Work out the finished part from the listing and answer in its coordinate system (mm). Face numbers are marked on the shaded views. A direction names the side the tool comes from. Coordinates: 2 decimals unless noted, no trailing zeros. Order: outer loops, then holes, each group sorted by start corner. A loop starts at its lowest first (then second) coordinate and runs counter-clockwise, first axis right, second up.
1. Find the intervals of material crossed by probe 1 along X at (y, z) = (104.5, 44.5); probe 2 along Y at (x, z) = (-40, -46); probe 3 along X at (y, z) = (10.5, 18.5), in increasing order.
2. The part is cut by section C-C, the plane x = 41. Give the vertices of the cut face in (y, z), then the cut area to 3 significant figures.
3. The part is cut by section B-B, the plane z = -39. Give the vertices of the cut face in (x, y), then the cut area to 3 significant figures.
4. A tool of negligible diameter and unlimited length cuts with its end or side. For the marked faces 4, 5, 6 and 7, from which of +Z, -Z, +X, -X, +Y, -Y can it reach the whole face along a straight path? Write none if from no direction.
5. Determine the mould class of the marked faces 1, 2 and 3 for opening direction X: +X half, -X half, draft (parallel to the pull), parting line (faces both ways), or undercut.
6. Flat-ended cylindrical pins translate along their axes: pin 1 Ø13 at (x, z) = (34.5, -22) entering from +Y; pin 2 Ø1 at (y, z) = (61, 24.5) entering from +X; pin 3 Ø10 at (y, z) = (75, 26) entering from -X. Find the tip coordinate at first contact, or state that the pin passes through.
7. The part is cut by section A-A, the plane y = 16.5. Give the vertices of the cut face in (x, z).
Autodesk Fusion 360 part; units mm, degrees
sketch "Esquisse1" plane through (0, 0, 0) normal (0, 0, 1) x (1, 0, 0)
  line L0 (0, 10) -> (-12.5, 10)
  line L1 (-12.5, 10) -> (-12.5, 110)
  line L2 (-12.5, 110) -> (-22.5, 110)
  line L3 (-22.5, 110) -> (-22.5, 10)
  line L4 (-22.5, 10) -> (-55.5, 10)
  line L5 (-55.5, 10) -> (-55.5, 0)
  line L6 (-55.5, 0) -> (0, 0)
  line L7 (0, 1.75) -> (0, 22.5)
  line L8 (1.75, 0) -> (22.5, 0)
  line L9 (0, 10) -> (12.5, 10)
  line L10 (12.5, 10) -> (12.5, 110)
  line L11 (12.5, 110) -> (22.5, 110)
  line L12 (22.5, 110) -> (22.5, 10)
  line L13 (22.5, 10) -> (55.5, 10)
  line L14 (55.5, 10) -> (55.5, 0)
  line L15 (55.5, 0) -> (0, 0)
  dimension "d13" = 12.5
  dimension "d15" = 10
  dimension "d16" = 10
  dimension "d17" = 100
  dimension "d19" = 10
  dimension "d20" = 55.5
extrude "Extrusion1" add sketch "Esquisse1" along normal mid plane 100
fillet "Congé5" radius 1.5 1 edges at (55.5, 10, 0)
fillet "Congé5" radius 1.5 1 edges at (-55.5, 10, 0)
fillet "Congé5" radius 1.5 1 edges at (12.5, 10, 0)
fillet "Congé5" radius 1.5 1 edges at (-12.5, 10, 0)
fillet "Congé5" radius 1.5 1 edges at (0, 10, -50)
fillet "Congé5" radius 1.5 1 edges at (0, 10, 50)
fillet "Congé6" radius 5 1 edges at (22.5, 10, 0)
fillet "Congé6" radius 5 1 edges at (-22.5, 10, 0)
fillet "Congé7" radius 1.5 5 edges at (-22.5, 62.5, 50) (-23.9645, 11.4645, 50) (-40.75, 10, 50) (-55.0607, 9.5607, 50) (-55.5, 4.25, 50)
fillet "Congé7" radius 1.5 5 edges at (22.5, 62.5, 50) (23.9645, 11.4645, 50) (40.75, 10, 50) (55.0607, 9.5607, 50) (55.5, 4.25, 50)
fillet "Congé7" radius 1.5 5 edges at (-55.5, 4.25, -50) (-55.0607, 9.5607, -50) (-40.75, 10, -50) (-23.9645, 11.4645, -50) (-22.5, 62.5, -50)
fillet "Congé7" radius 1.5 5 edges at (22.5, 62.5, -50) (23.9645, 11.4645, -50) (40.75, 10, -50) (55.0607, 9.5607, -50) (55.5, 4.25, -50)
fillet "Congé7" radius 1.5 1 edges at (17.5, 110, 50)
fillet "Congé7" radius 1.5 1 edges at (-17.5, 110, 50)
fillet "Congé7" radius 1.5 1 edges at (-17.5, 110, -50)
fillet "Congé7" radius 1.5 1 edges at (17.5, 110, -50)
fillet "Congé7" radius 1.5 4 edges at (22.5, 110, 0) (12.5, 110, 0) (-12.5, 110, 0) (-22.5, 110, 0)
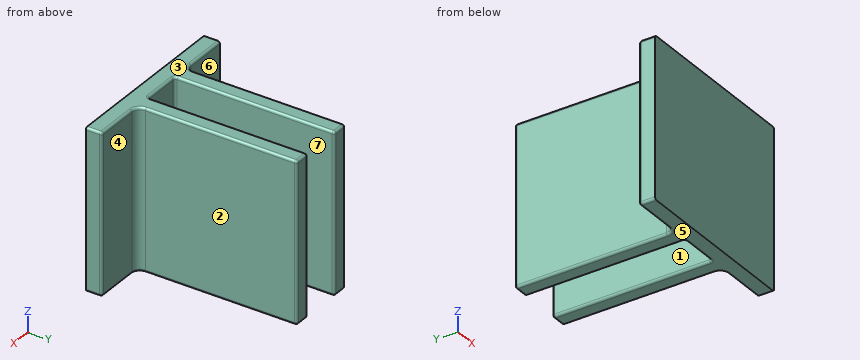
Geometry says:
1. probe 1: x = -22.5 to -12.5, 12.5 to 22.5
1. probe 2: y = 0 to 10
1. probe 3: x = -25.32 to -12.12, 12.12 to 25.32
2. outline: (0, -50) - (8.5, -50) arc R1.5 ccw to (10, -48.5) - (10, 48.5) arc R1.5 ccw to (8.5, 50) - (0, 50) - close
2. area: 999 mm2
3. outline: (-55.5, 0) - (55.5, 0) - (55.5, 8.5) arc R1.5 ccw to (54, 10) - (27.5, 10) arc R5 cw to (22.5, 15) - (22.5, 108.5) arc R1.5 ccw to (21, 110) - (14, 110) arc R1.5 ccw to (12.5, 108.5) - (12.5, 11.5) arc R1.5 cw to (11, 10) - (-11, 10) arc R1.5 cw to (-12.5, 11.5) - (-12.5, 108.5) arc R1.5 ccw to (-14, 110) - (-21, 110) arc R1.5 ccw to (-22.5, 108.5) - (-22.5, 15) arc R5 cw to (-27.5, 10) - (-54, 10) arc R1.5 ccw to (-55.5, 8.5) - close
3. area: 3,120 mm2
4. face 4: +Z, -Z, +X, +Y
4. face 5: -Z, +X, -X, +Y, -Y
4. face 6: +Z, -Z, -X, +Y
4. face 7: +Z, -Z, +Y
5. face 1: undercut
5. face 2: +X half
5. face 3: draft
6. pin 1: stops at y = 10
6. pin 2: stops at x = 22.5
6. pin 3: stops at x = -22.5
7. outline: (-22.5, -48.5) arc R1.5 ccw to (-21, -50) - (-14, -50) arc R1.5 ccw to (-12.5, -48.5) - (-12.5, 48.5) arc R1.5 ccw to (-14, 50) - (-21, 50) arc R1.5 ccw to (-22.5, 48.5) - close; (12.5, -48.5) arc R1.5 ccw to (14, -50) - (21, -50) arc R1.5 ccw to (22.5, -48.5) - (22.5, 48.5) arc R1.5 ccw to (21, 50) - (14, 50) arc R1.5 ccw to (12.5, 48.5) - close
